Autodesk Inventor part; units mm, degrees
ref_plane "YZ Plane" through (0, 0, 0) normal (1, 0, 0) x (0, 1, 0)
ref_plane "XZ Plane" through (0, 0, 0) normal (0, 1, 0) x (-1, 0, 0)
ref_plane "XY Plane" through (0, 0, 0) normal (0, 0, 1) x (1, 0, 0)
sketch "Sketch1" plane through (0, 0, 0) normal (0, 1, 0) x (-1, 0, 0)
  line L0 (-28.5, -57) -> (-28.5, -28.5) construction
  line L1 (-28.5, -28.5) -> (-57, -28.5) construction
  line L2 (0, -49) -> (-3, -49)
  line L3 (-3, -49) -> (-3, -57)
  line L4 (0, -49) -> (0, -39)
  line L5 (0, -39) -> (-3, -39)
  line L6 (-3, -39) -> (-3, -28.5)
  line L7 (0, -8) -> (-3, -8)
  line L8 (-3, -8) -> (-3, 0)
  line L9 (0, -18) -> (-3, -18)
  line L10 (-3, -18) -> (-3, -28.5)
  line L11 (0, -8) -> (0, -18)
  line L12 (0, -39) -> (0, -49)
  line L13 (0, -49) -> (0, -39)
  line L14 (0, -18) -> (0, -8)
  line L15 (-57, -49) -> (-54, -49)
  line L16 (-54, -49) -> (-54, -57)
  line L17 (-57, -49) -> (-57, -39)
  line L18 (-57, -39) -> (-54, -39)
  line L19 (-54, -39) -> (-54, -28.5)
  line L20 (-57, -8) -> (-54, -8)
  line L21 (-54, -8) -> (-54, 0)
  line L22 (-57, -18) -> (-54, -18)
  line L23 (-54, -18) -> (-54, -28.5)
  line L24 (-57, -8) -> (-57, -18)
  line L25 (-57, -39) -> (-57, -49)
  line L26 (-57, -49) -> (-57, -39)
  line L27 (-57, -18) -> (-57, -8)
  line L28 (-57, -49) -> (-57, -39)
  line L29 (-57, -18) -> (-57, -8)
  line L30 (-28.5, -54) -> (-36.5, -54)
  line L31 (-36.5, -54) -> (-36.5, -57)
  line L32 (-28.5, -54) -> (-20.5, -54)
  line L33 (-20.5, -54) -> (-20.5, -57)
  line L34 (-3, -57) -> (-20.5, -57)
  line L35 (-36.5, -57) -> (-54, -57)
  line L36 (-28.5, -3) -> (-36.5, -3)
  line L37 (-36.5, -3) -> (-36.5, 0)
  line L38 (-20.5, -3) -> (-20.5, 0)
  line L39 (-28.5, -3) -> (-20.5, -3)
  line L40 (-54, 0) -> (-36.5, 0)
  line L41 (-20.5, 0) -> (-3, 0)
  point P0 (0, 0)
  point P1 (0, -57)
  dimension "d3" = 3
  dimension "d4" = 10
  dimension "d5" = 3
  dimension "d6" = 3
  dimension "d7" = 8
extrude "Extrusion1" add sketch "Sketch1" along normal blind 3
sketch "Sketch2" plane through (0, 3, 0) normal (0, 1, 0) x (1, 0, 0)
  line L0 (36.5, 0) -> (54, 0)
  line L1 (36.5, 3) -> (36.5, 0)
  line L2 (36.5, 0) -> (36.5, 3)
  line L3 (36.5, 3) -> (54, 3)
  line L4 (54, 0) -> (54, 8)
  line L5 (20.5, 0) -> (20.5, 3)
  line L6 (20.5, 0) -> (20.5, 3)
  line L7 (20.5, 3) -> (36.5, 3)
  line L8 (20.5, 3) -> (36.5, 3)
  line L9 (36.5, 3) -> (36.5, 0)
  line L10 (3, 0) -> (20.5, 0)
  line L11 (20.5, 0) -> (20.5, 3)
  line L12 (3, 0) -> (3, 3)
  line L13 (3, 8) -> (3, 0)
  line L14 (20.5, 3) -> (3, 3)
  point P0 (0, 0)
extrude "Extrusion2" cut sketch "Sketch2" against normal up to surface (3 mm away)
sketch "Sketch3" plane through (0, 3, 0) normal (0, 1, 0) x (1, 0, 0)
  line L0 (3, 3) -> (20.5, 3)
  line L1 (3, 3) -> (54, 3)
  line L2 (20.5, 3) -> (20.5, 0)
  line L3 (36.5, 54) -> (20.5, 54)
  line L4 (28.5, 54) -> (28.5, 14.4088) construction
  line L5 (54, 3) -> (36.5, 3)
  line L6 (36.5, 3) -> (36.5, 0)
  line L7 (20.5, 0) -> (36.5, 0)
  point P0 (0, 0)
  dimension "d12" = 17.5
extrude "Extrusion3" add sketch "Sketch3" against normal up to surface (3 mm away)
sketch "Sketch4" plane through (0, 3, 0) normal (0, 1, 0) x (1, 0, 0)
  line L0 (36.5, 54) -> (20.5, 54)
  line L1 (20.5, 54) -> (3, 54)
  line L2 (3, 57) -> (3, 49)
  line L3 (36.5, 57) -> (36.5, 54)
  line L4 (36.5, 54) -> (54, 54)
  line L5 (54, 49) -> (54, 57)
  line L6 (20.5, 57) -> (3, 57)
  line L7 (3, 54) -> (3, 57)
  line L8 (3, 57) -> (20.5, 57)
  line L9 (20.5, 57) -> (20.5, 54)
  line L10 (36.5, 57) -> (36.5, 54)
  line L11 (54, 57) -> (36.5, 57)
  line L12 (36.5, 57) -> (54, 57)
  line L13 (54, 57) -> (54, 54)
  point P0 (0, 0)
extrude "Extrusion4" cut sketch "Sketch4" against normal up to surface (3 mm away)
sketch "Sketch5" plane through (0, 3, 0) normal (0, 1, 0) x (1, 0, 0)
  line L0 (54, 18) -> (54, 39)
  line L1 (54, 28.5) -> (3, 28.5) construction
  line L2 (3, 39) -> (3, 18)
  line L3 (3, 3) -> (20.5, 3)
  line L4 (3, 3) -> (20.5, 3)
  line L5 (20.5, 3) -> (20.5, 0)
  line L6 (20.5, 0) -> (36.5, 0)
  line L7 (20.5, 0) -> (36.5, 0)
  line L8 (36.5, 0) -> (36.5, 3)
  line L9 (36.5, 3) -> (54, 3)
  line L10 (36.5, 3) -> (54, 3)
  line L11 (3, 54) -> (20.5, 54)
  line L12 (20.5, 54) -> (20.5, 57)
  line L13 (20.5, 57) -> (36.5, 57)
  line L14 (36.5, 57) -> (36.5, 54)
  line L15 (36.5, 54) -> (54, 54)
  line L16 (20.5, 54) -> (36.5, 54)
  line L17 (54, 54) -> (3, 54)
  point P0 (0, 0)
extrude "Extrusion5" add sketch "Sketch5" against normal up to surface (3 mm away)
sketch "Sketch6" plane through (0, 3, 0) normal (0, 1, 0) x (1, 0, 0)
  line L0 (3, 39) -> (3, 18)
  line L1 (3, 28.5) -> (54, 28.5) construction
  line L2 (54, 18) -> (54, 39)
  circle A0 centre (28.5, 28.5) radius 2.55
  line L3 (18.9611, 22.4556) -> (18.9611, 35.5833) construction
  line L4 (18.9611, 35.5833) -> (23.3056, 35.5833) construction
  line L5 (23.3056, 35.5833) -> (23.3056, 22.4556) construction
  line L6 (23.3056, 22.4556) -> (18.9611, 22.4556) construction
  point P0 (0, 0)
  dimension "d19" = 5.1
extrude "Extrusion6" cut sketch "Sketch6" against normal up to surface (3 mm away)
properties part number "Superior"
Input: part model. Units: mm. Frame: model coordinates. A direction names the side the tool comes from. Give positions to 0.01 mm unless a question says otherwise; leave off trailing zeros. Order: outer loops, then holes, each group sorted by start corner. A loop starts at its lowest first (then second) coordinate and runs counter-clockwise, first axis right, second up. Notation, with made-up numbers: (16.25, 75.5) - (38.25, 75.5) arc R18 ccw to (38.25, 99.5) - close; hole circle Ø6 at (73.25, 34). An arc over 180 degrees is marked (long way). Answer as a JSON object with one key per item and string values. Group by question number.
Q1. First-contact query: pin 1 Ø1.5 at (x, y) = (55, 1.5) entering from -Z; pin 2 Ø3 at (x, z) = (28.5, -28.5) entering from +Y; pin 3 Ø0.9 at (x, y) = (1.5, 1.5) entering from +Z; pin 4 Ø0.9 at (y, z) = (1, -6.5) entering from -X. Flat tips, straight axial feed; report the tip coordinate or a pass-through.
Q2. Cut plane D-D, the plane x = 53. Output: boundary loops of the cut face in (y, z), then the cut area to 3 significant figures.
Q3. Cut plane A-A, the plane z = -28.5. Output: boundary loops of the cut face in (x, y).
Q4. Line query: probe 1 along Z at (x, y) = (28.5, 1.1); probe 2 along X at (y, z) = (2.2, -28.5); probe 3 along Z at (x, y) = (46.5, 1.35). Output: solid intervals per line, ascending.
Q5. Set-up query: faces 1 (the face through (1, 1, -18)), 2 (the face through (3, 1, -6)), 3 (the face through (56, 1, -39)). Return all of +Z, -Z, +X, -X, +Y, -Y with unobstructed straight access to the full face (end or side cutting, diameter ignored); none if empty.
Q6. Cut plane C-C, the plane x = 28.5. Output: boundary loops of the cut face in (y, z), then the cut area to 3 significant figures.
Results:
{
 "1": {"pin 1": "z = -49", "pin 2": "through", "pin 3": "z = -8", "pin 4": "x = 3"},
 "2": {"outline": "(0, -54) - (3, -54) - (3, -3) - (0, -3) - close", "area": "153 mm^2"},
 "3": {"outline": "(3, 0) - (25.95, 0) - (25.95, 3) - (3, 3) - close; (31.05, 0) - (54, 0) - (54, 3) - (31.05, 3) - close"},
 "4": {"probe 1": "-57 to -31.05, -25.95 to 0", "probe 2": "3 to 25.95, 31.05 to 54", "probe 3": "-54 to -3"},
 "5": {"face 1": "-X, +Y, -Y", "face 2": "+Z, -X, +Y, -Y", "face 3": "+X, +Y, -Y"},
 "6": {"outline": "(0, -57) - (3, -57) - (3, -31.05) - (0, -31.05) - close; (0, -25.95) - (3, -25.95) - (3, 0) - (0, 0) - close", "area": "156 mm^2"}
}
